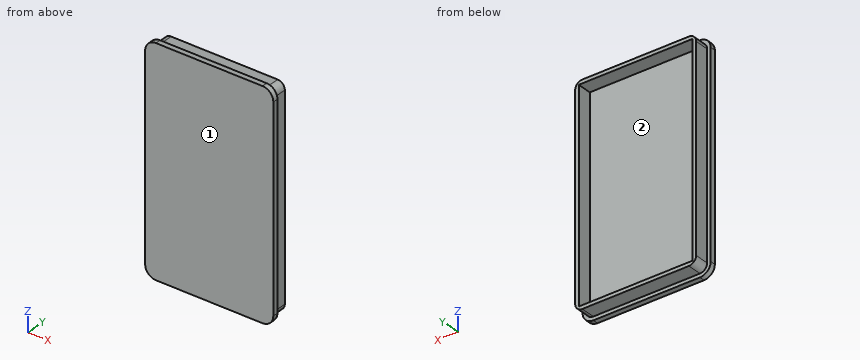
Autodesk Inventor part; units mm, degrees
ref_plane "YZ Plane" through (0, 0, 0) normal (1, 0, 0) x (0, 1, 0)
ref_plane "XZ Plane" through (0, 0, 0) normal (0, 1, 0) x (-1, 0, 0)
ref_plane "XY Plane" through (0, 0, 0) normal (0, 0, 1) x (1, 0, 0)
sketch "スケッチ1" plane through (0, 0, 0) normal (0, 1, 0) x (-1, 0, 0)
  line L0 (15.5, -28.5) -> (-15.5, -28.5)
  line L1 (-15.5, -28.5) -> (-15.5, 28.5)
  line L2 (-15.5, 28.5) -> (15.5, 28.5)
  line L3 (15.5, 28.5) -> (15.5, -28.5)
  line L4 (15.5, -28.5) -> (-15.5, 28.5) construction
  line L5 (-15.5, -28.5) -> (15.5, 28.5) construction
  line L6 (15.8, -28.8) -> (-15.8, -28.8)
  line L7 (-15.8, -28.8) -> (-15.8, 28.8)
  line L8 (-15.8, 28.8) -> (15.8, 28.8)
  line L9 (15.8, 28.8) -> (15.8, -28.8)
  line L10 (16.8, -29.8) -> (-16.8, -29.8)
  line L11 (-16.8, -29.8) -> (-16.8, 29.8)
  line L12 (-16.8, 29.8) -> (16.8, 29.8)
  line L13 (16.8, 29.8) -> (16.8, -29.8)
  line L14 (17.8, -30.8) -> (-17.8, -30.8)
  line L15 (-17.8, -30.8) -> (-17.8, 30.8)
  line L16 (-17.8, 30.8) -> (17.8, 30.8)
  line L17 (17.8, 30.8) -> (17.8, -30.8)
  point P0 (0, 0)
  dimension "d0" = 31
  dimension "d1" = 57
  dimension "d2" = 0.3
  dimension "d3" = 1
  dimension "d4" = 1
extrude "押し出し1" add sketch "スケッチ1" against normal blind 1.5 contours L0 L1 L2 L3 | L6 L7 L8 L9 | L10 L11 L12 L13 | L14 L15 L16 L17
extrude "押し出し2" add sketch "スケッチ1" along normal blind 4 contours L10 L11 L12 L13
fillet "フィレット1" radius 2 4 edges at (16.8, 2, 29.8) (16.8, 2, -29.8) (-16.8, 2, -29.8) (-16.8, 2, 29.8)
fillet "フィレット2" radius 3 4 edges at (-17.8, -0.75, 30.8) (-17.8, -0.75, -30.8) (17.8, -0.75, 30.8) (17.8, -0.75, -30.8)
sketch "スケッチ2" plane through (0, 0, 0) normal (0, 1, 0) x (1, 0, 0)
  point P0 (0, 0)
Part model, mm, in its own coordinate system. Face numbers are marked on the shaded views. Round coordinates to 2 decimals unless told otherwise and drop trailing zeros. Write each loop counter-clockwise with the first axis right and the second up, starting at its lowest first coordinate (ties: lowest second). Pieces come first, ordered by that corner, then holes. Notation, with made-up numbers: (34.25, -2) - (70.25, -2) arc R22 ccw to (70.25, 5) - close; hole circle Ø11 at (20, 50). An arc over 180 degrees is marked (long way). Use CSV: the item, a comma, the result in double quotes.
Item 1: Pull direction Z, two halves, no side cores. Call the marked faces 1 and 2: pulls with the +Z half, pulls with the -Z half, needs draft (parallel to the pull), parting line crosses it, or undercut.
Results list:
face 1,"needs draft"
face 2,"undercut"
Item 2: Slice it at A-A, the plane y = 1.25. Write the cut outline in (x, z), then the cut area to 3 significant figures.
Results list:
outline,"(-16.8, -27.8) arc R2 ccw to (-14.8, -29.8) - (14.8, -29.8) arc R2 ccw to (16.8, -27.8) - (16.8, 27.8) arc R2 ccw to (14.8, 29.8) - (-14.8, 29.8) arc R2 ccw to (-16.8, 27.8) - close; hole (-15.8, -28.8) - (15.8, -28.8) - (15.8, 28.8) - (-15.8, 28.8) - close"
area,"179 mm²"
Item 3: Flat gauge pins, fed straight in: P1, Ø2, axis at x = -6, y = 2, coming from the -Z side; P2, Ø3, axis at x = 3, y = 0.5, coming from the -Z side; P3, Ø9.5, axis at x = -4, z = -11.5, coming from the +Y side. Where does each tip first touch, or does it go through?
Results list:
P1,"stops at z = -29.8"
P2,"stops at z = -30.8"
P3,"stops at y = 0"
Item 4: Slice it at C-C, the plane x = -6. Write the cut outline in (y, z), then the cut area to 3 significant figures.
Results list:
outline,"(-1.5, -30.8) - (0, -30.8) - (0, -29.8) - (4, -29.8) - (4, -28.8) - (0, -28.8) - (0, 28.8) - (4, 28.8) - (4, 29.8) - (0, 29.8) - (0, 30.8) - (-1.5, 30.8) - close"
area,"100 mm²"
Item 5: Wall check: L1, parallel to Z at x = -3.5, y = 1.4; L2, parallel to X at y = 2.7, z = -6.5; L3, parallel to Y at x = 7, z = 24. Give the ranges that are in metal, low to high.
Results list:
L1,"z = -29.8 to -28.8, 28.8 to 29.8"
L2,"x = -16.8 to -15.8, 15.8 to 16.8"
L3,"y = -1.5 to 0"
Item 6: Slice it at B-B, the plane z = -21.5. Write the cut outline in (x, y), then the cut area to 3 significant figures.
Results list:
outline,"(-17.8, -1.5) - (17.8, -1.5) - (17.8, 0) - (16.8, 0) - (16.8, 4) - (15.8, 4) - (15.8, 0) - (-15.8, 0) - (-15.8, 4) - (-16.8, 4) - (-16.8, 0) - (-17.8, 0) - close"
area,"61.4 mm²"
